Check sheet for the drawn part. Datum: minimum x, y, z corner. Units: mm. A direction names the side the tool comes from. Give positions to 0.01 mm unless a question says otherwise; leave off trailing zeros. Order: outer loops, then holes, each group sorted by start corner. A loop starts at its lowest first (then second) coordinate and runs counter-clockwise, first axis right, second up. Notation, with made-up numbers: (-13, 64.25) -> (19, 64.25) arc R30 cw to (19, 86.25) -> close; hole circle Ø11 at (1, 47.25). An arc over 180 degrees is marked (long way). One line per question, with ' | ' between items. Start each with the question number.
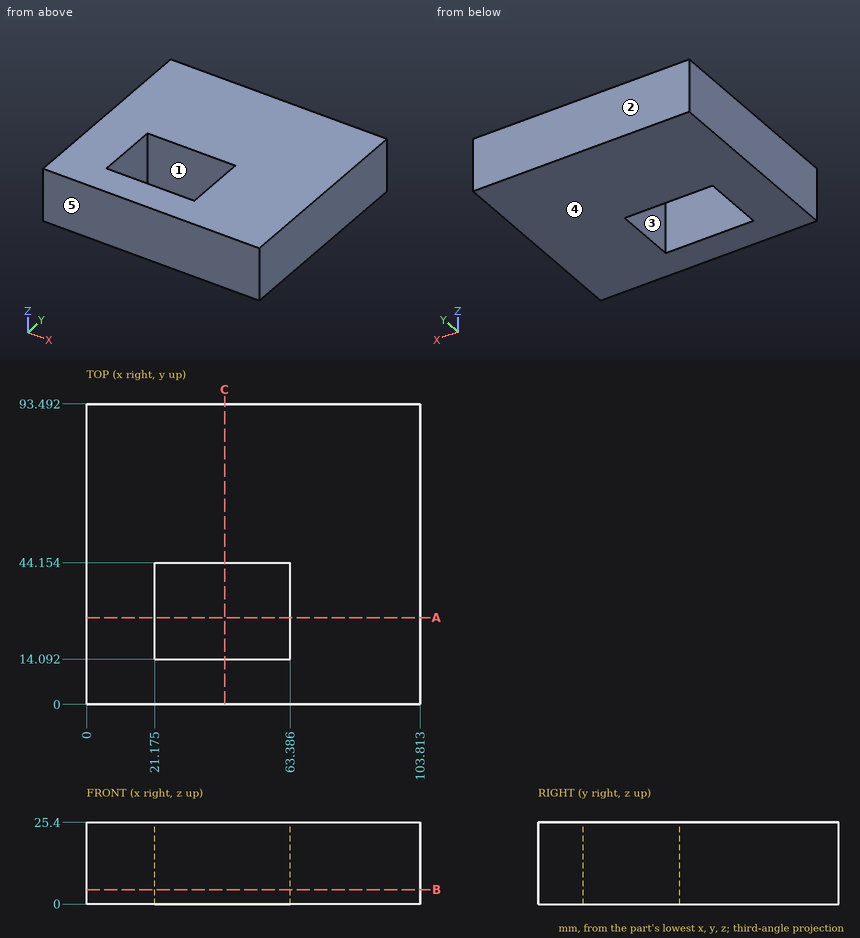
1. Tool access check on the marked faces 1 and 2. Record the directions out of +Z, -Z, +X, -X, +Y, -Y that give a thin tool (end or side, any length) a straight path to the whole face; none if there is none.
2. Scan lines: probe 1 along X at (y, z) = (34, 17.25) (1 decimal); probe 2 along Y at (x, z) = (26.5, 20.75) (1 decimal). Record each from-to range of solid material in increasing order.
3. Mould release check, pull along Y, two halves, no side actions. Record for the marked faces 3, 4 and 5: +Y half, -Y half, draft (parallel to the pull), parting line (faces both ways), or undercut.
4. Cross-section at C-C on x = 43. Record the boundary of the cut face in (y, z) (1 decimal).
5. Cross-section at A-A on y = 27. Record the boundary of the cut face in (x, z) (1 decimal).
6. Cross-section at B-B on z = 4.5. Record the boundary of the cut face in (x, y) (1 decimal).
Response values:
1) face 1: +Z, -Z | face 2: +Z, -Z, +X, -X, +Y
2) probe 1: x = 0 to 21.2, 63.4 to 103.8 | probe 2: y = 0 to 14.1, 44.2 to 93.5
3) face 3: undercut | face 4: draft | face 5: -Y half
4) outline: (0, 0) -> (14.1, 0) -> (14.1, 25.4) -> (0, 25.4) -> close; (44.2, 0) -> (93.5, 0) -> (93.5, 25.4) -> (44.2, 25.4) -> close
5) outline: (0, 0) -> (21.2, 0) -> (21.2, 25.4) -> (0, 25.4) -> close; (63.4, 0) -> (103.8, 0) -> (103.8, 25.4) -> (63.4, 25.4) -> close
6) outline: (0, 0) -> (103.8, 0) -> (103.8, 93.5) -> (0, 93.5) -> close; hole (21.2, 14.1) -> (63.4, 14.1) -> (63.4, 44.2) -> (21.2, 44.2) -> close
